CAD build for the part. Positions are in the model's coordinates, mm. A direction names the side the tool comes from. Give positions to 0.01 mm unless a question says otherwise; leave off trailing zeros. Write each loop counter-clockwise with the first axis right and the second up, starting at its lowest first coordinate (ties: lowest second). Pieces come first, ordered by that corner, then holes. Notation, with made-up numbers: (83, 22.25) - (93, 22.25) arc R31 cw to (93, 51.25) - close; hole circle Ø8 at (20.5, 27). An arc over 180 degrees is marked (long way). Answer as a JSON object with one key per item and string values.
from build123d import *

# Parameters (mm, degrees)
SKETCH1_W           = 15
SKETCH1_H           = 15
BOSS_EXTRUDE1_DEPTH = 50.8
SKETCH3_R           = 5.715
CUT_EXTRUDE1_DEPTH  = 44.704
SKETCH5_R           = 4.953
CUT_EXTRUDE3_DEPTH  = 16
LPATTERN1_COUNT     = 4
LPATTERN1_PITCH     = 12.7
SKETCH4_R           = 5.08
CUT_EXTRUDE5_DEPTH  = 6.096


with BuildPart() as part:
    # Sketch1 → Boss-Extrude1 (new body)
    with BuildSketch(Plane(origin=(0, 0, 0), x_dir=(0, 0, -1), z_dir=(1, 0, 0))):
        Rectangle(SKETCH1_W, SKETCH1_H)
    extrude(amount=-BOSS_EXTRUDE1_DEPTH)

    # Sketch3 → Cut-Extrude1 (cut)
    with BuildSketch(Plane.ZY.offset(48.26)):
        Circle(SKETCH3_R)
    extrude(amount=-CUT_EXTRUDE1_DEPTH, mode=Mode.SUBTRACT)

    # Sketch5 → Cut-Extrude3 (cut, through all)
    with BuildSketch(Plane(origin=(0, -7.5, 0), x_dir=(-1, 0, 0), z_dir=(0, -1, 0))):
        with Locations((43.863365925, 0)):
            Circle(SKETCH5_R)
    cut_extrude3 = extrude(amount=-CUT_EXTRUDE3_DEPTH, mode=Mode.SUBTRACT)

    # LPattern1: Cut-Extrude3 ×4
    with Locations(*[(i * LPATTERN1_PITCH, 0, 0) for i in range(1, LPATTERN1_COUNT)]):
        add(cut_extrude3, mode=Mode.SUBTRACT)

    # Sketch4 → Cut-Extrude5 (cut)
    with BuildSketch(Plane(origin=(0, 0, 0), x_dir=(0, 0, -1), z_dir=(1, 0, 0))):
        Circle(SKETCH4_R)
    extrude(amount=-CUT_EXTRUDE5_DEPTH, mode=Mode.SUBTRACT)


solid = part.part
(1) Saw through at C-C, the plane z = 0. State how many separate pieces and enclosed holes the cut face has, and give its area (3 significant figures).
Answer key:
{"separate pieces": "9", "enclosed holes": "0", "area": "63.6 mm²"}
(2) 3-axis set-ups, long thin cutter, end or side, ignore diameter. For faces 1 (the face through (-26.22, -5.07, 2.64)), 2 (the face through (-25, -7.5, 0)), 3 (the face through (-1.36, -1.95, -4.69)): which of +Z, -Z, +X, -X, +Y, -Y reach the whole face in a straight line?
Answer key:
{"face 1": "none", "face 2": "+Z, -Z, +X, -X, -Y", "face 3": "+X"}
(3) Saw through at A-A, the plane y = 0. Give the cut face in (x, z) (3 decimals).
Answer key:
{"outline": "(-50.8, -7.5) - (0, -7.5) - (0, -5.08) - (-3.556, -5.08) - (-3.556, -5.715) - (-48.26, -5.715) - (-48.26, -2.281) arc R4.953 cw to (-48.26, 2.281) - (-48.26, 5.715) - (-3.556, 5.715) - (-3.556, 5.08) - (0, 5.08) - (0, 7.5) - (-50.8, 7.5) - close"}
(4) Saw through at B-B, the plane x = -5. Give the cut face in (y, z) (3 decimals).
Answer key:
{"outline": "(-7.5, -7.5) - (7.5, -7.5) - (7.5, -4.894) - (2.952, -4.894) arc R5.715 cw to (-2.952, -4.894) - (-7.5, -4.894) - close; (-7.5, 4.894) - (-2.952, 4.894) arc R5.715 cw to (2.952, 4.894) - (7.5, 4.894) - (7.5, 7.5) - (-7.5, 7.5) - close"}
(5) Pull direction X, two halves, no side cores. Call faces 4 (the face through (0, 5, 2)), 5 (the face through (-48.26, 0, -4)), 6 (the face through (-25, 0, 7.5)): pulls with the +X half, pulls with the -X half, needs draft (parallel to the pull), parting line crosses it, or undercut.
Answer key:
{"face 4": "pulls with the +X half", "face 5": "undercut", "face 6": "needs draft"}
(6) Flat gauge pin, fed straight in: P1, Ø1, axis at y = -2, z = 4, coming from the +X side. Where does the tip first touch, or does it go through?
Answer key:
{"P1": "stops at x = -48.26"}
(7) Saw through at D-D, the plane x = -41. Give the cut face in (y, z) (3 decimals).
Answer key:
{"outline": "(-7.5, -7.5) - (7.5, -7.5) - (7.5, -4.041) - (4.041, -4.041) arc R5.715 cw to (-4.041, -4.041) - (-7.5, -4.041) - close; (-7.5, 4.041) - (-4.041, 4.041) arc R5.715 cw to (4.041, 4.041) - (7.5, 4.041) - (7.5, 7.5) - (-7.5, 7.5) - close"}
(8) Probe L1, parallel to Z at x = -20.5, y = 0 (3 decimals); L2, parallel to X at y = 6.75, z = -3.75; L3, parallel to Z at x = -20, y = -7. List the from-to ranges inside material, lowest first. Write a range as [from, to].
Answer key:
{"L1": "z = [-7.5, -5.715], [5.715, 7.5]", "L2": "x = [-50.8, -47.1], [-40.63, -34.4], [-27.93, -21.7], [-15.23, -9], [-2.53, 0]", "L3": "z = [-7.5, -4.71], [4.71, 7.5]"}
